from build123d import *

# Parameters (mm, degrees)
SKETCH_1_R          = 6
EXTRUDE_1_DEPTH     = 1
SKETCH_2_R          = 4
EXTRUDE_2_DEPTH     = 4
SKETCH_3_R          = 2.05
CUT_EXTRUDE_1_DEPTH = 10.848857802
CHAMFER_1_SIZE      = 0.2


with BuildPart() as part:
    # 草图1 → 凸台-拉伸1 (new body)
    with BuildSketch(Plane.XY):
        Circle(SKETCH_1_R)
    extrude(amount=EXTRUDE_1_DEPTH)

    # 草图2 → 凸台-拉伸2 (add)
    with BuildSketch(Plane.XY.offset(1)):
        Circle(SKETCH_2_R)
    extrude(amount=EXTRUDE_2_DEPTH)

    # 草图3 → 切除-拉伸1 (cut, through all)
    with BuildSketch(Plane.XY.offset(5)):
        Circle(SKETCH_3_R)
    extrude(amount=-CUT_EXTRUDE_1_DEPTH, mode=Mode.SUBTRACT)

    # 倒角1
    chamfer_1_edges = [part.edges().sort_by_distance(p)[0] for p in [
        (-2.05, 0, 0),
        (-2.05, 0, 5),
        (-4, 0, 5),
    ]]
    chamfer(chamfer_1_edges, length=CHAMFER_1_SIZE)


solid = part.part
Check sheet for the modelled part. Datum: model origin and axes. Units: mm. A direction names the side the tool comes from. Round coordinates to 2 decimals unless told otherwise and drop trailing zeros. Order: outer loops, then holes, each group sorted by start corner. A loop starts at its lowest first (then second) coordinate and runs counter-clockwise, first axis right, second up.
Q1. Set-up check for faces 4 (the face through (3, 0, 0)), 5 (the face through (-0.867, -3.905, 2.873)): record each of +Z, -Z, +X, -X, +Y, -Y from which the full face is reachable in a straight line by a thin tool's end or side.
Filled sheet:
face 4: -Z, +X, -X, +Y, -Y
face 5: +Z
Q2. Depth check by flat-ended pin: P1, Ø2.5, axis at x = 0, y = 0, coming from the -Z side; P2, Ø3, axis at y = -4, z = 4, coming from the -X side. Enter the tip coordinate at first touch or a pass-through.
Filled sheet:
P1: passes through
P2: stops at x = -3.12
Q3. Cross-section at A-A, the plane x = 0. Enter the section's corners in (y, z).
Filled sheet:
outline: (-6, 0) - (-2.25, 0) - (-2.05, 0.2) - (-2.05, 4.8) - (-2.25, 5) - (-3.8, 5) - (-4, 4.8) - (-4, 1) - (-6, 1) - close; (2.05, 0.2) - (2.25, 0) - (6, 0) - (6, 1) - (4, 1) - (4, 4.8) - (3.8, 5) - (2.25, 5) - (2.05, 4.8) - close
Q4. Cross-section at D-D, the plane x = 5. Enter the section's corners in (y, z).
Filled sheet:
outline: (-3.32, 0) - (3.32, 0) - (3.32, 1) - (-3.32, 1) - close
Q5. Draft check along Y on faces 1 (the face through (-1.42, -3.92, 1)), 2 (the face through (-5.994, 0.264, 0.493)), 3 (the face through (-0.267, 2.033, 2.532)). Enter one of: pulls with the +Y half, pulls with the -Y half, needs draft (parallel to the pull), parting line crosses it, or undercut.
Filled sheet:
face 1: needs draft
face 2: parting line crosses it
face 3: undercut
Q6. Scan lines: L1, parallel to Y at x = 0, z = 1.2; L2, parallel to Z at x = 4.5, y = -2.25; L3, parallel to Y at x = -1.75, z = 0.85. Record each from-to range of solid material in increasing order.
Filled sheet:
L1: y = -4 to -2.05, 2.05 to 4
L2: z = 0 to 1
L3: y = -5.74 to -1.07, 1.07 to 5.74
Q7. Cross-section at C-C, the plane z = 3.3. Enter the section's corners in (x, y).
Filled sheet:
outline: circle Ø8 at (0, 0); hole circle Ø4.1 at (0, 0)
